```python
from build123d import *

# Parameters (mm, degrees)
F0_R     = 3.5
F0_R_2   = 2
F1_DEPTH = 15
F2_R     = 2.45
F2_R_2   = 2
F3_DEPTH = 1
F4_R     = 2.91
F4_R_2   = 2
F5_DEPTH = 7


with BuildPart() as f1:
    # F0 (on Top) → F1 (new body)
    with BuildSketch(Plane.XY):
        Circle(F0_R)
        Circle(F0_R_2, mode=Mode.SUBTRACT)
    extrude(amount=F1_DEPTH)

    # F2 (on Top) → F3 (join)
    with BuildSketch(Plane.XY):
        Circle(F2_R)
        Circle(F2_R_2, mode=Mode.SUBTRACT)
    extrude(amount=-F3_DEPTH)

    # F4 (on face) → F5 (join)
    with BuildSketch(Plane(origin=(0, 0, -1), x_dir=(1, 0, 0), z_dir=(0, 0, -1))):
        Circle(F4_R)
        Circle(F4_R_2, mode=Mode.SUBTRACT)
    extrude(amount=F5_DEPTH)


solid = f1.part
```
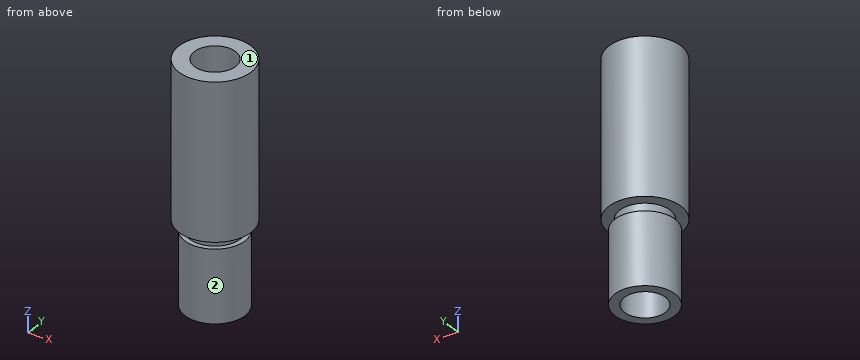
The listing builds one solid part. Answer for the finished solid, in the listing's coordinates (mm). Face numbers are marked on the shaded views. A direction names the side the tool comes from. Give positions to 0.01 mm unless a question says otherwise; leave off trailing zeros. Loops run counter-clockwise (first coordinate to the right, second up) from the corner with the lowest first, then second, coordinate; pieces in that order, holes last. Notation, with made-up numbers: (-20, -13) - (39, -13) arc R19 cw to (39, 2) - close; hole circle Ø8 at (34, -25). An arc over 180 degrees is marked (long way). Return JSON: item names as keys, results as strings. Group by question number.
1. Find section A-A (y = 0). Write down the section's boundary in (x, z), then the cut area to 3 significant figures.
2. Find section D-D (z = -5.5). Write down the section's boundary in (x, y), then the cut area to 3 significant figures.
3. Which of the six approach directions +Z, -Z, +X, -X, +Y, -Y give full straight-line access (tool end or side, diameter ignored) to the marked faces 1 and 2?
4. Straight lines are drawn through the part: line 1 (Z direction, x = 2.5, y = 0); line 2 (Y direction, x = 0, z = 3.5); line 3 (Y direction, x = 0, z = -0.65). For each, find the intervals that lie inside material, in ascending order. Write a range as [from, to].
5. Given pin 1 Ø3 at (x, z) = (2.5, 0) entering from +Y; pin 2 Ø1 at (x, z) = (-2, 8.5) entering from +Y; pin 3 Ø3.5 at (x, y) = (0, 0) entering from +Z; pin 4 Ø3 at (x, z) = (2, 7) entering from +Y, each flat-ended and moving along its own axis, determine where each tip first touches the part or whether it passes through.
6. Find section C-C (z = 12.75). Write down the section's boundary in (x, y), then the cut area to 3 significant figures.
Verdict:
{
 "1": {"outline": "(-3.5, 0) - (-2.45, 0) - (-2.45, -1) - (-2.91, -1) - (-2.91, -8) - (-2, -8) - (-2, 15) - (-3.5, 15) - close; (2, -8) - (2.91, -8) - (2.91, -1) - (2.45, -1) - (2.45, 0) - (3.5, 0) - (3.5, 15) - (2, 15) - close", "area": "58.6 mm^2"},
 "2": {"outline": "circle Ø5.82 at (0, 0); hole circle Ø4 at (0, 0)", "area": "14.0 mm^2"},
 "3": {"face 1": "+Z, +X, -X, +Y, -Y", "face 2": "-Z"},
 "4": {"line 1": "z = [-8, -1], [0, 15]", "line 2": "y = [-3.5, -2], [2, 3.5]", "line 3": "y = [-2.45, -2], [2, 2.45]"},
 "5": {"pin 1": "stops at y = 3.35", "pin 2": "stops at y = 3.16", "pin 3": "passes through", "pin 4": "stops at y = 3.46"},
 "6": {"outline": "circle Ø7 at (0, 0); hole circle Ø4 at (0, 0)", "area": "25.9 mm^2"}
}
